from build123d import *

# Parameters (mm, degrees)
F0_R          = 5
F1_DEPTH      = 25
F1_DEPTH_BACK = 25
F2_DEPTH      = 2
F2_DEPTH_BACK = 2
F3_DEPTH      = 2


with BuildPart() as f1:
    # F0 (on Front) → F1 (new body, two sides)
    with BuildSketch(Plane.XZ) as f1_sk:
        with Locations((45.321487, 23.518129)):
            Circle(F0_R)
    extrude(amount=F1_DEPTH)
    extrude(f1_sk.sketch, amount=-F1_DEPTH_BACK)

    # F0 (on Front) → F2 (join, two sides)
    with BuildSketch(Plane.XZ) as f2_sk:
        with BuildLine():
            Line((145.381006, 69.213781), (134.997648, 67.769526))
            ThreePointArc((134.997648, 67.769526), (133.089386, 71.443028), (131.030724, 75.034405))
            Line((131.030724, 75.034405), (137.859376, 82.988619))
            Line((137.859376, 82.988619), (127.787244, 80.081359))
            ThreePointArc((127.787244, 80.081359), (125.375611, 83.445896), (122.826797, 86.70774))
            Line((122.826797, 86.70774), (128.45394, 95.55281))
            Line((128.45394, 95.55281), (118.898074, 91.241727))
            ThreePointArc((118.898074, 91.241727), (116.032165, 94.228807), (113.045085, 97.094717))
            Line((113.045085, 97.094717), (117.356168, 106.650582))
            Line((117.356168, 106.650582), (108.511098, 101.023439))
            ThreePointArc((108.511098, 101.023439), (105.249254, 103.572253), (101.884716, 105.983886))
            Line((101.884716, 105.983886), (104.791977, 116.056018))
            Line((104.791977, 116.056018), (96.837763, 109.227366))
            ThreePointArc((96.837763, 109.227366), (93.246386, 111.286028), (89.572883, 113.19429))
            Line((89.572883, 113.19429), (91.017138, 123.577649))
            Line((91.017138, 123.577649), (84.115706, 115.6865))
            ThreePointArc((84.115706, 115.6865), (80.267905, 117.213102), (76.36022, 118.579147))
            Line((76.36022, 118.579147), (76.312068, 129.062356))
            Line((76.312068, 129.062356), (70.60391, 120.269352))
            ThreePointArc((70.60391, 120.269352), (66.578016, 121.232816), (62.515697, 122.028835))
            Line((62.515697, 122.028835), (60.976119, 132.398488))
            Line((60.976119, 132.398488), (56.577436, 122.882628))
            ThreePointArc((56.577436, 122.882628), (52.455405, 123.263341), (48.321149, 123.473129))
            Line((48.321149, 123.473129), (45.321487, 133.518129))
            Line((45.321487, 133.518129), (42.321824, 123.473129))
            ThreePointArc((42.321824, 123.473129), (38.187569, 123.263341), (34.065537, 122.882628))
            Line((34.065537, 122.882628), (29.666855, 132.398488))
            Line((29.666855, 132.398488), (28.127277, 122.028835))
            ThreePointArc((28.127277, 122.028835), (24.064958, 121.232816), (20.039064, 120.269352))
            Line((20.039064, 120.269352), (14.330906, 129.062356))
            Line((14.330906, 129.062356), (14.282754, 118.579147))
            ThreePointArc((14.282754, 118.579147), (10.375069, 117.213102), (6.527268, 115.6865))
            Line((6.527268, 115.6865), (-0.374165, 123.577649))
            Line((-0.374165, 123.577649), (1.07009, 113.19429))
            ThreePointArc((1.07009, 113.19429), (-2.603412, 111.286028), (-6.194789, 109.227366))
            Line((-6.194789, 109.227366), (-14.149003, 116.056018))
            Line((-14.149003, 116.056018), (-11.241743, 105.983886))
            ThreePointArc((-11.241743, 105.983886), (-14.60628, 103.572253), (-17.868124, 101.023439))
            Line((-17.868124, 101.023439), (-26.713194, 106.650582))
            Line((-26.713194, 106.650582), (-22.402111, 97.094717))
            ThreePointArc((-22.402111, 97.094717), (-25.389191, 94.228807), (-28.255101, 91.241727))
            Line((-28.255101, 91.241727), (-37.810966, 95.55281))
            Line((-37.810966, 95.55281), (-32.183823, 86.70774))
            ThreePointArc((-32.183823, 86.70774), (-34.732637, 83.445896), (-37.14427, 80.081359))
            Line((-37.14427, 80.081359), (-47.216402, 82.988619))
            Line((-47.216402, 82.988619), (-40.38775, 75.034405))
            ThreePointArc((-40.38775, 75.034405), (-42.446412, 71.443028), (-44.354674, 67.769526))
            Line((-44.354674, 67.769526), (-54.738033, 69.213781))
            Line((-54.738033, 69.213781), (-46.846884, 62.312348))
            ThreePointArc((-46.846884, 62.312348), (-48.373486, 58.464547), (-49.739531, 54.556862))
            Line((-49.739531, 54.556862), (-60.22274, 54.50871))
            Line((-60.22274, 54.50871), (-51.429736, 48.800552))
            ThreePointArc((-51.429736, 48.800552), (-52.3932, 44.774658), (-53.189219, 40.712339))
            ThreePointArc((-53.189219, 40.712339), (-53.660657, 37.749613), (-54.043012, 34.774078))
            ThreePointArc((-54.043012, 34.774078), (-54.423725, 30.652047), (-54.633513, 26.517792))
            Line((-54.633513, 26.517792), (-64.678513, 23.518129))
            Line((-64.678513, 23.518129), (-54.633513, 20.518467))
            ThreePointArc((-54.633513, 20.518467), (-54.423725, 16.384211), (-54.043012, 12.26218))
            Line((-54.043012, 12.26218), (-63.558872, 7.863497))
            Line((-63.558872, 7.863497), (-53.189219, 6.323919))
            ThreePointArc((-53.189219, 6.323919), (-52.3932, 2.2616), (-51.429736, -1.764294))
            Line((-51.429736, -1.764294), (-60.22274, -7.472452))
            Line((-60.22274, -7.472452), (-49.739531, -7.520604))
            ThreePointArc((-49.739531, -7.520604), (-48.373486, -11.428289), (-46.846884, -15.27609))
            Line((-46.846884, -15.27609), (-54.738033, -22.177522))
            Line((-54.738033, -22.177522), (-44.354674, -20.733268))
            ThreePointArc((-44.354674, -20.733268), (-42.446412, -24.40677), (-40.38775, -27.998147))
            Line((-40.38775, -27.998147), (-47.216402, -35.952361))
            Line((-47.216402, -35.952361), (-37.14427, -33.0451))
            ThreePointArc((-37.14427, -33.0451), (-34.732637, -36.409638), (-32.183823, -39.671482))
            Line((-32.183823, -39.671482), (-37.810966, -48.516552))
            Line((-37.810966, -48.516552), (-28.255101, -44.205469))
            ThreePointArc((-28.255101, -44.205469), (-25.389191, -47.192549), (-22.402111, -50.058458))
            Line((-22.402111, -50.058458), (-26.713194, -59.614324))
            Line((-26.713194, -59.614324), (-17.868124, -53.987181))
            ThreePointArc((-17.868124, -53.987181), (-14.60628, -56.535995), (-11.241743, -58.947628))
            Line((-11.241743, -58.947628), (-14.149003, -69.01976))
            Line((-14.149003, -69.01976), (-6.194789, -62.191108))
            ThreePointArc((-6.194789, -62.191108), (-2.603412, -64.24977), (1.07009, -66.158032))
            Line((1.07009, -66.158032), (-0.374165, -76.54139))
            Line((-0.374165, -76.54139), (6.527268, -68.650242))
            ThreePointArc((6.527268, -68.650242), (10.375069, -70.176843), (14.282754, -71.542889))
            Line((14.282754, -71.542889), (14.330906, -82.026098))
            Line((14.330906, -82.026098), (20.039064, -73.233094))
            ThreePointArc((20.039064, -73.233094), (24.064958, -74.196558), (28.127277, -74.992577))
            Line((28.127277, -74.992577), (29.666855, -85.36223))
            Line((29.666855, -85.36223), (34.065537, -75.84637))
            ThreePointArc((34.065537, -75.84637), (38.187569, -76.227082), (42.321824, -76.436871))
            Line((42.321824, -76.436871), (45.321487, -86.481871))
            Line((45.321487, -86.481871), (48.321149, -76.436871))
            ThreePointArc((48.321149, -76.436871), (52.455405, -76.227082), (56.577436, -75.84637))
            Line((56.577436, -75.84637), (60.976119, -85.36223))
            Line((60.976119, -85.36223), (62.515697, -74.992577))
            ThreePointArc((62.515697, -74.992577), (66.578016, -74.196558), (70.60391, -73.233094))
            Line((70.60391, -73.233094), (76.312068, -82.026098))
            Line((76.312068, -82.026098), (76.36022, -71.542889))
            ThreePointArc((76.36022, -71.542889), (80.267905, -70.176843), (84.115706, -68.650242))
            Line((84.115706, -68.650242), (91.017138, -76.54139))
            Line((91.017138, -76.54139), (89.572883, -66.158032))
            ThreePointArc((89.572883, -66.158032), (93.246386, -64.24977), (96.837763, -62.191108))
            Line((96.837763, -62.191108), (104.791977, -69.01976))
            Line((104.791977, -69.01976), (101.884716, -58.947628))
            ThreePointArc((101.884716, -58.947628), (105.249254, -56.535995), (108.511098, -53.987181))
            Line((108.511098, -53.987181), (117.356168, -59.614324))
            Line((117.356168, -59.614324), (113.045085, -50.058458))
            ThreePointArc((113.045085, -50.058458), (116.032165, -47.192549), (118.898074, -44.205469))
            Line((118.898074, -44.205469), (128.45394, -48.516552))
            Line((128.45394, -48.516552), (122.826797, -39.671482))
            ThreePointArc((122.826797, -39.671482), (125.375611, -36.409638), (127.787244, -33.0451))
            Line((127.787244, -33.0451), (137.859376, -35.952361))
            Line((137.859376, -35.952361), (131.030724, -27.998147))
            ThreePointArc((131.030724, -27.998147), (133.089386, -24.40677), (134.997648, -20.733268))
            Line((134.997648, -20.733268), (145.381006, -22.177522))
            Line((145.381006, -22.177522), (137.489858, -15.27609))
            ThreePointArc((137.489858, -15.27609), (139.016459, -11.428289), (140.382504, -7.520604))
            Line((140.382504, -7.520604), (150.865714, -7.472452))
            Line((150.865714, -7.472452), (142.07271, -1.764294))
            ThreePointArc((142.07271, -1.764294), (143.036173, 2.2616), (143.832193, 6.323919))
            Line((143.832193, 6.323919), (154.201845, 7.863497))
            Line((154.201845, 7.863497), (144.685986, 12.26218))
            ThreePointArc((144.685986, 12.26218), (145.066698, 16.384211), (145.276487, 20.518467))
            Line((145.276487, 20.518467), (155.321487, 23.518129))
            Line((155.321487, 23.518129), (145.276487, 26.517792))
            ThreePointArc((145.276487, 26.517792), (145.066698, 30.652047), (144.685986, 34.774078))
            Line((144.685986, 34.774078), (154.201845, 39.172761))
            Line((154.201845, 39.172761), (143.832193, 40.712339))
            ThreePointArc((143.832193, 40.712339), (143.036173, 44.774658), (142.07271, 48.800552))
            Line((142.07271, 48.800552), (150.865714, 54.50871))
            Line((150.865714, 54.50871), (140.382504, 54.556862))
            ThreePointArc((140.382504, 54.556862), (139.016459, 58.464547), (137.489858, 62.312348))
            Line((137.489858, 62.312348), (145.381006, 69.213781))
        make_face()
        with Locations((45.321487, 23.518129)):
            Circle(F0_R, mode=Mode.SUBTRACT)
    extrude(amount=F2_DEPTH)
    extrude(f2_sk.sketch, amount=-F2_DEPTH_BACK)

    # F0 (on Front) → F3 (join, through all)
    with BuildSketch(Plane.XZ):
        with BuildLine():
            Line((-53.189219, 40.712339), (-63.558872, 39.172761))
            Line((-63.558872, 39.172761), (-54.043012, 34.774078))
            ThreePointArc((-54.043012, 34.774078), (-53.660657, 37.749613), (-53.189219, 40.712339))
        make_face()
    extrude(amount=-F3_DEPTH)


solid = f1.part
Verification items for the finished model (mm, model axes). A direction names the side the tool comes from. Coordinates: 2 decimals unless noted, no trailing zeros. Order: outer loops, then holes, each group sorted by start corner. A loop starts at its lowest first (then second) coordinate and runs counter-clockwise, first axis right, second up. Notation, with made-up numbers: M -10.75,-27.75 L 18.25,-27.75 A30 ccw 18.25,5.25 Z; hole C 67.25,72 d10. An arc over 180 degrees is marked long. One line per item, written item: value. Start each with the question number.
Item 1: Gauge pin test, flat ends, axial feed: pin 1 (10 mm diameter, centred on x = 47, y = -9.5, fed in from -Z); pin 2 (1.5 mm diameter, centred on y = -2.5, z = 7.5, fed in from +X); pin 3 (4 mm diameter, centred on x = 96.5, z = 111, fed in from +Y). Record the tip position at first contact, or that the pin passes through.
Item 2: Mould release check, pull along X, two halves, no side actions. Record for faces 1 (the flat face through (125.68, -0.03, -44.16)), 2 (the flat face through (73.5, -0.03, 124.73)), 3 (the flat face through (-55.888, -0.028, 51.695)), 4 (the flat face through (87.52, -0.03, -72.54)): released by +X, released by -X, zero draft, split by the parting line, or undercut.
Item 3: Sectioned sample at B-B (z = 72.5). Enter the section's corners in (x, y).
Item 4: Access from +Z, -Z, +X, -X, +Y, -Y to the whole of each face (thin tool, end or side, straight path). Record for faces 5 (the flat face through (113, -0.03, 103.88)), 6 (the cylindrical face through (50.09, -13.66, 25.02)), 7 (the cylindrical face through (50.09, 13.34, 25.02)), 8 (the cylindrical face through (-25.35, -0.03, 94.27)).
Item 5: Sectioned sample at A-A (y = 20.5). Enter the section's corners in (x, z).
Item 6: Sectioned sample at C-C (z = 44.5). Enter the section's corners in (x, y).
Item 7: Scan lines: probe 1 along Y at (x, z) = (-14, 102); probe 2 along X at (y, z) = (-1.5, 64); probe 3 along X at (y, z) = (19, 23). Record each from-to range of solid material in increasing order.
Conclusion:
1. pin 1: stops at z = 18.52
1. pin 2: stops at x = 154.2
1. pin 3: stops at y = 2
2. face 1: released by +X
2. face 2: undercut
2. face 3: released by -X
2. face 4: undercut
3. outline: M -41.86,-2 L 132.5,-2 L 132.5,2 L -41.86,2 Z
4. face 5: +Z, +Y, -Y
4. face 6: -Y
4. face 7: +Y
4. face 8: +Y, -Y
5. outline: C 45.32,23.52 d10
6. outline: M -52.45,-2 L 143.1,-2 L 143.1,2 L -52.45,2 Z
7. probe 1: y = -2 to 2
7. probe 2: x = -48.78 to 139.42
7. probe 3: x = 40.35 to 50.29
